```python
from build123d import *

# Parameters (mm, degrees)
F1_W     = 112
F1_H     = 34.5
F2_DEPTH = 3
F0_W     = 5
F0_H     = 15
F0_W_2   = 16.181867
F0_H_2   = 5
F3_DEPTH = 5
F4_R     = 1.5
F5_DEPTH = 25
F6_R     = 1
F7_SIZE  = 5


with BuildPart() as f2:
    # F1 (on Top) → F2 (new body)
    with BuildSketch(Plane.XY):
        with Locations((-11.597955, 10.057821)):
            Rectangle(F1_W, F1_H)
    extrude(amount=F2_DEPTH)

    # F0 (on Top) → F3 (join)
    with BuildSketch(Plane.XY):
        with Locations((-65.097955, 10.307821)):
            Rectangle(F0_W, F0_H)
        with Locations((-11.597955, 10.307821)):
            Rectangle(F0_W, F0_H)
        with Locations((41.902045, 10.307821)):
            Rectangle(F0_W, F0_H)
        with Locations((-39.348996, 24.807821)):
            Rectangle(F0_W_2, F0_H_2)
        with Locations((-39.348996, -4.692179)):
            Rectangle(F0_W_2, F0_H_2)
        with Locations((13.451004, 24.807821)):
            Rectangle(F0_W_2, F0_H_2)
        with Locations((13.451004, -4.692179)):
            Rectangle(F0_W_2, F0_H_2)
    extrude(amount=-F3_DEPTH)

    # F4 (on face) → F5 (cut)
    with BuildSketch(Plane(origin=(0, 0, -5), x_dir=(1, 0, 0), z_dir=(0, 0, -1))):
        with Locations((-65.097955, -10.307821)):
            Circle(F4_R)
        with Locations((-11.597955, -10.307821)):
            Circle(F4_R)
        with Locations((41.902045, -10.307821)):
            Circle(F4_R)
        with Locations((-39.258062, 5.192179)):
            Circle(F4_R)
        with Locations((13.541938, 5.192179)):
            Circle(F4_R)
        with Locations((13.541938, -25.307821)):
            Circle(F4_R)
        with Locations((-39.258062, -25.307821)):
            Circle(F4_R)
    extrude(amount=-F5_DEPTH, mode=Mode.SUBTRACT)

    # F6
    f6_edges = [f2.edges().sort_by_distance(p)[0] for p in [
        (-62.597955, 2.807821, -2.5),
        (-62.597955, 17.807821, -2.5),
        (-47.439929, -2.192179, -2.5),
        (-31.258062, -2.192179, -2.5),
        (-47.439929, 22.307821, -2.5),
        (-31.258062, 22.307821, -2.5),
        (-14.097955, 17.807821, -2.5),
        (-14.097955, 2.807821, -2.5),
        (5.360071, -2.192179, -2.5),
        (21.541938, -2.192179, -2.5),
        (39.402045, 2.807821, -2.5),
        (-9.097955, 2.807821, -2.5),
        (-9.097955, 17.807821, -2.5),
        (39.402045, 17.807821, -2.5),
        (21.541938, 22.307821, -2.5),
        (5.360071, 22.307821, -2.5),
    ]]
    fillet(f6_edges, radius=F6_R)

    # F7
    f7_edges = [f2.edges().sort_by_distance(p)[0] for p in [
        (-67.597955, 27.307821, 1.5),
        (44.402045, 27.307821, 1.5),
        (44.402045, -7.192179, 1.5),
        (-67.597955, -7.192179, 1.5),
    ]]
    chamfer(f7_edges, length=F7_SIZE)


solid = f2.part
```
Geometry: final body of the model. Coordinates: model frame, mm. A direction names the side the tool comes from. Coordinates: 2 decimals unless noted, no trailing zeros. Write each loop counter-clockwise with the first axis right and the second up, starting at its lowest first coordinate (ties: lowest second). Pieces come first, ordered by that corner, then holes. Notation, with made-up numbers: M 72.25,-18.5 L 121.25,-18.5 A22 cw 121.25,17.5 Z; hole C -37.5,17.25 d4. An arc over 180 degrees is marked long. Use CSV: the item, a comma, the result in double quotes. Start each with the question number.
1. Mould query, pull axis X, two halves, no side actions, for faces 1 (the face through (-39, 22.308, -2)), 2 (the face through (40.403, 10.242, -1.056)), 3 (the face through (41.94, 24.77, 1.48)), 4 (the face through (-14.098, 10, -2)). Classes: pulls with the +X half, pulls with the -X half, needs draft (parallel to the pull), parting line crosses it, or undercut.
2. Ray query, probe 1 along X at (y, z) = (6.5, -0.75); probe 2 along X at (y, z) = (25, 2.5); probe 3 along X at (y, z) = (23.5, -1). Return the intervals inside material, ascending.
3. Cut plane C-C on z = -2.25. Count the separate pieces of the cut face and the enclosed holes in it, plus the area to 3 significant figures.
4. Cut plane A-A on x = 10. Return the cut outline in (y, z), plus the area to 4 significant figures.
5. Cut plane B-B on y = 5.5. Return the cut outline in (x, z).
6. First-contact query: P1, Ø1.2, axis at y = -4.5, z = -2, coming from the -X side; P2, Ø1.2, axis at x = 42.5, z = -3, coming from the -Y side; P3, Ø12, axis at x = -54, y = 5.5, coming from the -Z side. Flat tips, straight axial feed; report the tip coordinate or a pass-through.
7. Cut plane D-D on x = 30.5. Return the cut outline in (y, z).
8. Reachability of faces 5 (the face through (-66, 2.808, -2)), 6 (the face through (13, 22.308, -2)), 7 (the face through (5.36, -5, -2)), 8 (the face through (-66, 17.808, -2)), 9 (the face through (21.542, -5, -2)) from +Z, -Z, +X, -X, +Y, -Y: full face, straight path, thin tool, end or side. Return the list, or none.
Entries:
1,face 1,"needs draft"
1,face 2,"undercut"
1,face 3,"pulls with the +X half"
1,face 4,"undercut"
2,probe 1,"-67.6 to -62.6, -14.1 to -9.1, 39.4 to 44.4"
2,probe 2,"-64.91 to -40.73, -37.79 to 12.07, 15.01 to 41.71"
2,probe 3,"-47.44 to -31.26, 5.36 to 21.54"
3,separate pieces,"7"
3,enclosed holes,"7"
3,area,"496 mm²"
4,outline,"M -7.19,-5 L -2.19,-5 L -2.19,0 L 22.31,0 L 22.31,-5 L 27.31,-5 L 27.31,3 L -7.19,3 Z"
4,area,"153.5 mm²"
5,outline,"M -67.6,-5 L -62.6,-5 L -62.6,0 L -14.1,0 L -14.1,-5 L -9.1,-5 L -9.1,0 L 39.4,0 L 39.4,-5 L 44.4,-5 L 44.4,3 L -67.6,3 Z"
6,P1,"x = -47.44"
6,P2,"y = 2.81"
6,P3,"z = 0"
7,outline,"M -7.19,0 L 27.31,0 L 27.31,3 L -7.19,3 Z"
8,face 5,"-Z, +X, -X, -Y"
8,face 6,"-Z, +X, -X"
8,face 7,"-Z, +Y, -Y"
8,face 8,"-Z, +X, -X, +Y"
8,face 9,"-Z, +X, +Y, -Y"
